Can you work these out from the model? Positions are in its coordinate system, mm. Coordinates: 2 decimals unless noted, no trailing zeros. Loops run counter-clockwise (first coordinate to the right, second up) from the corner with the lowest first, then second, coordinate; pieces in that order, holes last. Notation, with made-up numbers: M 4.5,44.5 L 61.5,44.5 A13 ccw 61.5,58.5 Z; hole C -12.5,86 d5. An arc over 180 degrees is marked long. Answer as a JSON object with one key per item and string values. Group by question number.
Item 1: If I drill on line 1 (X direction, y = 25, z = 694) (3 decimals); line 2 (Y direction, x = 25, z = 475.5) (3 decimals), over which ranges is the centre line in solid material (lowest first)?
Item 2: Suppose I cut it at C-C (y = 22). Write out the boundary of the cut face in (x, z) (3 decimals), then the cut area to 3 significant figures.
Item 3: Suppose I cut it at A-A (z = 156). Write out the boundary of the cut face in (x, y) (3 decimals).
Item 4: Suppose I cut it at B-B (x = 64). Write out the boundary of the cut face in (y, z) (3 decimals), then the cut area to 3 significant figures.
Autodesk Inventor part; units mm, degrees
ref_plane "YZ Plane" through (0, 0, 0) normal (1, 0, 0) x (0, 1, 0)
ref_plane "XZ Plane" through (0, 0, 0) normal (0, 1, 0) x (-1, 0, 0)
ref_plane "XY Plane" through (0, 0, 0) normal (0, 0, 1) x (1, 0, 0)
sketch "Sketch1" plane through (0, 0, 0) normal (0, 0, 1) x (1, 0, 0)
  line L0 (0, 0) -> (101.6, 0)
  line L1 (101.6, 0) -> (101.6, 50.8)
  line L2 (101.6, 50.8) -> (0, 50.8)
  line L3 (0, 50.8) -> (0, 0)
  dimension "d0" = 101.6
  dimension "d1" = 50.8
extrude "Extrusion1" add sketch "Sketch1" along normal blind 1219.2
shell "Shell1" thickness 3.175 removed faces 2 at (67.7333, 16.9333, 0) at (67.7333, 16.9333, 1219.2)
fillet "Fillet1" radius 3.175 8 edges at (0, 50.8, 609.6) (3.175, 3.175, 609.6) (98.425, 3.175, 609.6) (3.175, 47.625, 609.6) (98.425, 47.625, 609.6) (101.6, 50.8, 609.6) (0, 0, 609.6) (101.6, 0, 609.6)
properties part number "2x3_Tube"
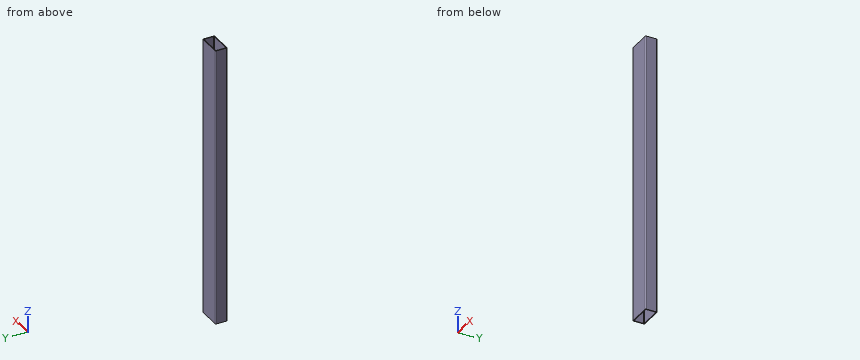
From the geometry:
{
 "1": {"line 1": "0 to 3.175, 98.425 to 101.6", "line 2": "0 to 3.175, 47.625 to 50.8"},
 "2": {"outline": "M 0,0 L 3.175,0 L 3.175,1219.2 L 0,1219.2 Z; M 98.425,0 L 101.6,0 L 101.6,1219.2 L 98.425,1219.2 Z", "area": "7,740 mm2"},
 "3": {"outline": "M 0,3.175 A3.175 ccw 3.175,0 L 98.425,0 A3.175 ccw 101.6,3.175 L 101.6,47.625 A3.175 ccw 98.425,50.8 L 3.175,50.8 A3.175 ccw 0,47.625 Z; hole M 3.175,6.35 A3.175 ccw 6.35,3.175 L 95.25,3.175 A3.175 ccw 98.425,6.35 L 98.425,44.45 A3.175 ccw 95.25,47.625 L 6.35,47.625 A3.175 ccw 3.175,44.45 Z"},
 "4": {"outline": "M 0,0 L 3.175,0 L 3.175,1219.2 L 0,1219.2 Z; M 47.625,0 L 50.8,0 L 50.8,1219.2 L 47.625,1219.2 Z", "area": "7,740 mm2"}
}
